```python
from build123d import *

# Parameters (mm, degrees)
SKETCH1_R         = 10.4521
SKETCH1_R_2       = 4.9276
BASE_DEPTH        = 1.1938
SKETCH2_R         = 9.6393
SKETCH2_R_2       = 8.89
TRACK_DEPTH       = 0.7112
SKETCH3_R         = 1.9431
PLATFORM_1_DEPTH  = 0.3302
SKETCH4_R         = 1.4859
SKETCH4_R_2       = 0.9779
PLATFORM_2_DEPTH  = 3.175
SKETCH5_R         = 0.9906
SKETCH5_R_2       = 0.7366
PLATFORM_3_DEPTH  = 1.9812
CIRPATTERN1_COUNT = 3


with BuildPart() as part:
    # Sketch1 → Base (new body)
    with BuildSketch(Plane.XY):
        Circle(SKETCH1_R)
        Circle(SKETCH1_R_2, mode=Mode.SUBTRACT)
    extrude(amount=BASE_DEPTH)

    # Sketch2 → Track (add)
    with BuildSketch(Plane(origin=(0, 0, 0), x_dir=(-1, 0, 0), z_dir=(0, 0, -1))):
        Circle(SKETCH2_R)
        Circle(SKETCH2_R_2, mode=Mode.SUBTRACT)
    extrude(amount=TRACK_DEPTH)

    # Sketch3 → Platform 1 (add)
    with BuildSketch(Plane.XY.offset(1.1938)):
        with Locations((0, 8.128)):
            Circle(SKETCH3_R)
        with Locations((0, -7.62)):
            Circle(SKETCH3_R)
    platform_1 = extrude(amount=PLATFORM_1_DEPTH)

    # Sketch4 → Platform 2 (add)
    with BuildSketch(Plane.XY.offset(1.524)):
        with Locations((0, 8.128)):
            Circle(SKETCH4_R)
        with Locations((0, -7.62)):
            Circle(SKETCH4_R_2)
    platform_2 = extrude(amount=PLATFORM_2_DEPTH)

    # Sketch5 → Platform 3 (add)
    with BuildSketch(Plane.XY.offset(4.699)):
        with Locations((0, 8.128)):
            Circle(SKETCH5_R)
        with Locations((0, -7.62)):
            Circle(SKETCH5_R_2)
    platform_3 = extrude(amount=PLATFORM_3_DEPTH)

    # CirPattern1: Platform 1, Platform 2, Platform 3 ×3 about axis
    cirpattern1_axis = Axis((0, 0, 0), (0, 0, 1))
    for i in range(1, CIRPATTERN1_COUNT):
        add(platform_1.rotate(cirpattern1_axis, i * 360 / CIRPATTERN1_COUNT))
        add(platform_2.rotate(cirpattern1_axis, i * 360 / CIRPATTERN1_COUNT))
        add(platform_3.rotate(cirpattern1_axis, i * 360 / CIRPATTERN1_COUNT))


solid = part.part
```
Could you check a few things on this model? Use its own coordinates, in mm. A direction names the side the tool comes from. Round coordinates to 2 decimals unless told otherwise and drop trailing zeros. Loops run counter-clockwise (first coordinate to the right, second up) from the corner with the lowest first, then second, coordinate; pieces in that order, holes last. Notation, with made-up numbers: (66.25, 41.5) - (81.25, 41.5) arc R23 ccw to (81.25, 57.5) - close; hole circle Ø2 at (-10.75, 77). An arc over 180 degrees is marked (long way). Answer in a Markdown table with one row per item. Add a question column.
(1) If we section it at D-D (y = -7.62): Please give me the cut outline in (x, z).
(2) I need wall thicknesses on line 1 along Y through (x, z) = (0, -0.45); line 2 along Y through (x, z) = (0, 4.25); line 3 along Z through (x, y) = (6.75, 0.5). Which ranges of each line are inside material? Lowest first, please.
(3) If we section it at B-B (z = 0.5): Please give me the cut outline in (x, y), plus the area to 3 significant figures.
(4) If we section it at A-A (y = 0): Please give me the cut outline in (x, z), plus the area to 3 significant figures.
(5) If we mould it in two halves opening along Y, with no side actions, what happens to faces 1 (the face through (-0.42, 6.23, 1.36)), 2 (the face through (0, 8, 6.68)), 3 (the face through (2.09, -9.41, -0.35))? For each: pulls with the +Y half, pulls with the -Y half, needs draft (parallel to the pull), parting line crosses it, or undercut.
(6) If we section it at C-C (x = 2.75): Please give me the cut outline in (y, z).
(7) For faces 4 (the face through (7, -4, 6.68)), 5 (the face through (6.05, -4.02, 5.68)), which set-ups out of +Z, -Z, +X, -X, +Y, -Y let a thin tool reach every point of the face, with its end or its side?
(8) I'm going to push flat-ended pins straight in: pin 1 (5.5 mm diameter, centred on x = 0.5, y = -4.5, fed in from -Z); pin 2 (1 mm diameter, centred on y = -3.5, z = 0.5, fed in from -X); pin 3 (2 mm diameter, centred on y = 6.5, z = 5, fed in from -X); pin 4 (6 mm diameter, centred on x = 0, y = 0, fed in from -Z). Where does each tip first touch, or does it pass through?
Model answer:
| question | item | result |
|---|---|---|
| 1 | outline | (-7.15, 0) - (-5.9, 0) - (-5.9, -0.71) - (-4.58, -0.71) - (-4.58, 0) - (4.58, 0) - (4.58, -0.71) - (5.9, -0.71) - (5.9, 0) - (7.15, 0) - (7.15, 1.19) - (1.94, 1.19) - (1.94, 1.52) - (0.98, 1.52) - (0.98, 4.7) - (0.74, 4.7) - (0.74, 6.68) - (-0.74, 6.68) - (-0.74, 4.7) - (-0.98, 4.7) - (-0.98, 1.52) - (-1.94, 1.52) - (-1.94, 1.19) - (-7.15, 1.19) - close |
| 2 | line 1 | y = -9.64 to -8.89, 8.89 to 9.64 |
| 2 | line 2 | y = -8.6 to -6.64, 6.64 to 9.61 |
| 2 | line 3 | z = 0 to 1.19 |
| 3 | outline | circle Ø20.9 at (0, 0); hole circle Ø9.86 at (0, 0) |
| 3 | area | 267 mm² |
| 4 | outline | (-10.45, 0) - (-9.64, 0) - (-9.64, -0.71) - (-8.89, -0.71) - (-8.89, 0) - (-4.93, 0) - (-4.93, 1.19) - (-10.45, 1.19) - close; (4.93, 0) - (8.89, 0) - (8.89, -0.71) - (9.64, -0.71) - (9.64, 0) - (10.45, 0) - (10.45, 1.19) - (4.93, 1.19) - close |
| 4 | area | 14.3 mm² |
| 5 | face 1 | undercut |
| 5 | face 2 | needs draft |
| 5 | face 3 | parting line crosses it |
| 6 | outline | (-10.08, 0) - (-9.24, 0) - (-9.24, -0.71) - (-8.45, -0.71) - (-8.45, 0) - (-4.09, 0) - (-4.09, 1.19) - (-10.08, 1.19) - close; (4.09, 0) - (8.45, 0) - (8.45, -0.71) - (9.24, -0.71) - (9.24, 0) - (10.08, 0) - (10.08, 1.19) - (4.09, 1.19) - close |
| 7 | face 4 | +Z, +X, -X, +Y, -Y |
| 7 | face 5 | +Z |
| 8 | pin 1 | stops at z = 0 |
| 8 | pin 2 | stops at x = -10.01 |
| 8 | pin 3 | stops at x = -1.32 |
| 8 | pin 4 | passes through |
